Build history of the part. All positions in model axes, mm. Face numbers are marked on the shaded views. A direction names the side the tool comes from. Give positions to 0.01 mm unless a question says otherwise; leave off trailing zeros. Order: outer loops, then holes, each group sorted by start corner. A loop starts at its lowest first (then second) coordinate and runs counter-clockwise, first axis right, second up. Notation, with made-up numbers: (-38.5, 88) -> (-13.5, 88) arc R20 ccw to (-13.5, 121) -> close; hole circle Ø1 at (76.25, 24.5). An arc over 180 degrees is marked (long way). Write item = value, one per line. Start each with the question number.
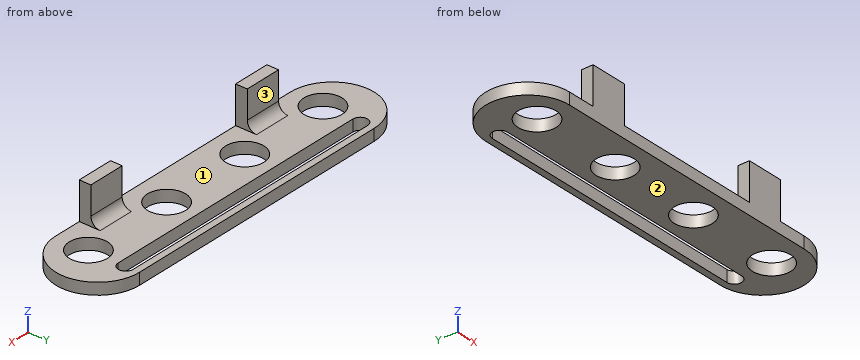
from build123d import *

# Parameters (mm, degrees)
SKETCH1_R           = 5.207
BOSS_EXTRUDE1_DEPTH = 3.175
SKETCH2_W           = 10.16
SKETCH2_H           = 3.175
BOSS_EXTRUDE2_DEPTH = 10.16
FILLET1_R           = 2.54
CUT_EXTRUDE2_REACH  = 53.837


with BuildPart() as part:
    # Sketch1 → Boss-Extrude1 (new body)
    with BuildSketch(Plane.XY):
        with BuildLine():
            Line((-38.1, 11.43), (38.1, 11.43))
            ThreePointArc((38.1, 11.43), (49.53, 0), (38.1, -11.43))
            Line((38.1, -11.43), (-38.1, -11.43))
            ThreePointArc((-38.1, -11.43), (-49.53, 0), (-38.1, 11.43))
        make_face()
        with Locations((-38.1, -2.54)):
            Circle(SKETCH1_R, mode=Mode.SUBTRACT)
        with Locations((-12.7, -2.54)):
            Circle(SKETCH1_R, mode=Mode.SUBTRACT)
        with Locations((12.7, -2.54)):
            Circle(SKETCH1_R, mode=Mode.SUBTRACT)
        with Locations((38.1, -2.54)):
            Circle(SKETCH1_R, mode=Mode.SUBTRACT)
    extrude(amount=BOSS_EXTRUDE1_DEPTH)

    # Sketch2 → Boss-Extrude2 (add)
    with BuildSketch(Plane.XY.offset(3.175)):
        with Locations((-25.4, -9.8425)):
            Rectangle(SKETCH2_W, SKETCH2_H)
        with Locations((25.4, -9.8425)):
            Rectangle(SKETCH2_W, SKETCH2_H)
    extrude(amount=BOSS_EXTRUDE2_DEPTH)

    # Fillet1
    fillet1_edges = [part.edges().sort_by_distance(p)[0] for p in [
        (25.4, -8.255, 3.175),
        (-25.4, -8.255, 3.175),
    ]]
    fillet(fillet1_edges, radius=FILLET1_R)

    # Sketch4 → Cut-Extrude2 (cut, up to next)
    with BuildSketch(Plane.XY.offset(3.175), mode=Mode.PRIVATE) as cut_extrude2_sk1:
        with BuildLine():
            Line((-38.1, 9.652), (38.1, 9.652))
            ThreePointArc((38.1, 9.652), (40.132, 7.62), (38.1, 5.588))
            Line((38.1, 5.588), (-38.1, 5.588))
            ThreePointArc((-38.1, 5.588), (-40.132, 7.62), (-38.1, 9.652))
        make_face()
    cut_extrude2_tool1 = extrude(cut_extrude2_sk1.sketch, amount=-CUT_EXTRUDE2_REACH, mode=Mode.PRIVATE) & part.part
    add(cut_extrude2_tool1.solids().sort_by_distance((0, 7.62, 3.175))[0], mode=Mode.SUBTRACT)


solid = part.part
(1) Flat gauge pins, fed straight in: P1, Ø4.5, axis at y = -7.5, z = 7, coming from the +X side; P2, Ø4, axis at x = -11, y = 4.5, coming from the +Z side (3 decimals); P3, Ø3, axis at y = -4.5, z = 1.5, coming from the +X side; P4, Ø9.5, axis at x = 12.7, y = -2.54, coming from the +Z side. Where does each tip first touch, or does it go through?
(2) Wall check: line 1 (Y direction, x = 38.1, z = 1.45); line 2 (Y direction, x = -28, z = 3); line 3 (Z direction, x = -3, y = -7.75) (3 decimals). Give the ranges that are in metal, low to high. Write a range as [from, to].
(3) Cut at D-D, the plane y = -2.54. Give the cut face in (x, z) (3 decimals).
(4) Cut at B-B, the plane x = -29. Give the cut face in (y, z) (3 decimals).
(5) 3-axis set-ups, long thin cutter, end or side, ignore diameter. For the marked faces 1, 2 and 3: which of +Z, -Z, +X, -X, +Y, -Y reach the whole face in a straight line?
(6) Cut at C-C, the plane z = 9. Give the cut face in (x, y) (3 decimals).
(7) Cut at A-A, the plane x = 12.7. Give the cut face in (y, z) (3 decimals), plus the area to 3 significant figures.
Results:
q1.P1 = 30.48
q1.P2 = 3.175
q1.P3 = 49.13
q1.P4 = through
q2.line_1 = [-11.43, -7.75], [2.67, 5.59], [9.65, 11.43]
q2.line_2 = [-11.43, 5.59], [9.65, 11.43]
q2.line_3 = [0, 3.175]
q3.outline = (-49.244, 0) -> (-43.307, 0) -> (-43.307, 3.175) -> (-49.244, 3.175) -> close; (-32.893, 0) -> (-17.907, 0) -> (-17.907, 3.175) -> (-32.893, 3.175) -> close; (-7.493, 0) -> (7.493, 0) -> (7.493, 3.175) -> (-7.493, 3.175) -> close; (17.907, 0) -> (32.893, 0) -> (32.893, 3.175) -> (17.907, 3.175) -> close; (43.307, 0) -> (49.244, 0) -> (49.244, 3.175) -> (43.307, 3.175) -> close
q4.outline = (-11.43, 0) -> (5.588, 0) -> (5.588, 3.175) -> (-5.715, 3.175) arc R2.54 cw to (-8.255, 5.715) -> (-8.255, 13.335) -> (-11.43, 13.335) -> close; (9.652, 0) -> (11.43, 0) -> (11.43, 3.175) -> (9.652, 3.175) -> close
q5.face_1 = +Z, +Y
q5.face_2 = -Z, +X, -X, +Y, -Y
q5.face_3 = +Z, +X, -X, +Y
q6.outline = (-30.48, -11.43) -> (-20.32, -11.43) -> (-20.32, -8.255) -> (-30.48, -8.255) -> close; (20.32, -11.43) -> (30.48, -11.43) -> (30.48, -8.255) -> (20.32, -8.255) -> close
q7.outline = (-11.43, 0) -> (-7.747, 0) -> (-7.747, 3.175) -> (-11.43, 3.175) -> close; (2.667, 0) -> (5.588, 0) -> (5.588, 3.175) -> (2.667, 3.175) -> close; (9.652, 0) -> (11.43, 0) -> (11.43, 3.175) -> (9.652, 3.175) -> close
q7.area = 26.6 mm2
